```python
from build123d import *

# Parameters (mm, degrees)
SKETCH1_R                      = 20.125
BOSS_EXTRUDE1_DEPTH            = 20
SKETCH12_W                     = 21.496046148
SKETCH12_H                     = 21.496046148
CUT_EXTRUDE1_DEPTH             = 15
CUT_EXTRUDE2_START             = -18
SKETCH16_R                     = 20.125
SKETCH16_R_2                   = 19.3
CUT_EXTRUDE2_DEPTH             = 18
FILLET3_R                      = 2
M5_CLEARANCE_HOLE1_D           = 5.5
M5_CLEARANCE_HOLE1_CSINK_D     = 5.55
M5_CLEARANCE_HOLE1_CSINK_ANGLE = 90


with BuildPart() as part:
    # Sketch1 → Boss-Extrude1 (new body)
    with BuildSketch(Plane(origin=(0, 0, 0), x_dir=(1, 0, 0), z_dir=(0, 1, 0))):
        with Locations(Location((0, 0, 0), (0, 0, 270))):
            Circle(SKETCH1_R)
    extrude(amount=BOSS_EXTRUDE1_DEPTH)

    # Sketch12 → Cut-Extrude1 (cut)
    with BuildSketch(Plane.XZ):
        Rectangle(SKETCH12_W, SKETCH12_H)
    extrude(amount=-CUT_EXTRUDE1_DEPTH, mode=Mode.SUBTRACT)

    # Sketch16 → Cut-Extrude2 (cut)
    with BuildSketch(Plane(origin=(0, 20, 0), x_dir=(1, 0, 0), z_dir=(0, 1, 0)).offset(CUT_EXTRUDE2_START)):
        with Locations(Location((0, 0, 0), (0, 0, 270))):
            Circle(SKETCH16_R)
        with Locations(Location((0, 0, 0), (0, 0, 270))):
            Circle(SKETCH16_R_2, mode=Mode.SUBTRACT)
    extrude(amount=CUT_EXTRUDE2_DEPTH, mode=Mode.SUBTRACT)

    # Fillet3
    # the kernel refuses this fillet: 2 mm, written as the material it takes off along each edge
    with BuildSketch(Plane(origin=(0, 20, 0), x_dir=(0, 0, 1), z_dir=(-1, 0, 0))) as fillet3_piece_1:
        with BuildLine():
            CenterArc((19.3 - FILLET3_R, -FILLET3_R), FILLET3_R, 0, 90)
            Line((19.3 - FILLET3_R, 0), (19.3 - FILLET3_R, FILLET3_R * 0.02))
            Line((19.3 - FILLET3_R, FILLET3_R * 0.02), (19.3 + FILLET3_R * 0.02, FILLET3_R * 0.02))
            Line((19.3 + FILLET3_R * 0.02, FILLET3_R * 0.02), (19.3 + FILLET3_R * 0.02, -FILLET3_R))
            Line((19.3 + FILLET3_R * 0.02, -FILLET3_R), (19.3, -FILLET3_R))
        make_face()
    revolve(axis=Axis((0, 20, 0), (0, 1, 0)), mode=Mode.SUBTRACT)
    with BuildSketch(Plane(origin=(0, 2, 0), x_dir=(0, 0, 1), z_dir=(-1, 0, 0))) as fillet3_piece_2:
        with BuildLine():
            CenterArc((18.125, -1.618448331), FILLET3_R, 0, 54.020199403)
            Line((19.3, 0), (19.3235, 0.032368967))
            ThreePointArc((19.3235, 0.032368967), (19.7125, 0.04), (20.125, 0.04))
            Line((20.125, 0.04), (20.165, 0))
            Line((20.165, 0), (20.165, -1.618448331))
            Line((20.165, -1.618448331), (20.125, -1.618448331))
        make_face()
    revolve(axis=Axis((0, 2, 0), (0, 1, 0)), mode=Mode.SUBTRACT)

    # M5 Clearance Hole1 (through all)
    with Locations(Plane(origin=(0, 20, 0), x_dir=(1, 0, 0), z_dir=(0, 1, 0))):
        with Locations((0, 0)):
            CounterSinkHole(M5_CLEARANCE_HOLE1_D / 2, M5_CLEARANCE_HOLE1_CSINK_D / 2, counter_sink_angle=M5_CLEARANCE_HOLE1_CSINK_ANGLE)


solid = part.part
```
The listing builds one solid part. Answer for the finished solid, in the listing's coordinates (mm). A direction names the side the tool comes from. Coordinates: 2 decimals unless noted, no trailing zeros. Loops run counter-clockwise (first coordinate to the right, second up) from the corner with the lowest first, then second, coordinate; pieces in that order, holes last. Notation, with made-up numbers: M -1,42.5 L 40,42.5 A28 ccw 40,73.5 Z; hole C 60.25,-7.5 d5. An arc over 180 degrees is marked long. Answer as a JSON object with one key per item and string values. Group by question number.
Item 1: Section B-B (x = 0) is taken. Write down the section's boundary in (y, z) (3 decimals), and give its area (3 significant figures).
Item 2: Each of these flat-tipped pins is pushed along its axis until it touches: P1, Ø5, axis at x = 7.5, y = 5.5, coming from the +Z side; P2, Ø12, axis at y = 5.5, z = 1, coming from the +X side (3 decimals); P3, Ø3, axis at y = 15, z = 15, coming from the +X side. Where does it stop, or does it pass through?
Item 3: Determine the mould class of faces 1 (the face through (-10.748, 7, 0)), 2 (the face through (0, 20, 4)), 3 (the face through (10.748, 7, 0)), 4 (the face through (6.045, 0.188, 19.196)) for opening direction Z: +Z half, -Z half, draft (parallel to the pull), parting line (faces both ways), or undercut.
Item 4: Section D-D (y = 15.75) is taken. Write down the section's boundary in (x, z), and give its area (3 significant figures).
Item 5: Consider L1, parallel to X at y = 8, z = 0.5; L2, parallel to X at y = 10.75, z = 2; L3, parallel to Y at x = 10, z = -4. Determine where each line is inside the solid, lowest interval first.
Item 6: Section A-A (z = 0) is taken. Write down the section's boundary in (x, y) (3 decimals).
Item 7: Which of the six approach directions +Z, -Z, +X, -X, +Y, -Y give full straight-line access (tool end or side, diameter ignored) to faces 5 (the face through (0.596, 17.453, 2.685)), 6 (the face through (0, 7, 10.748)), 7 (the face through (19.136, 9.888, -2.512))?
Item 8: Section C-C (y = 9) is taken. Write down the section's boundary in (x, z), and give its area (3 significant figures).
Solved:
{
 "1": {"outline": "M 0,-20.125 L 0.382,-20.125 A2 ccw 2,-19.3 L 18,-19.3 A2 ccw 20,-17.3 L 20,-2.775 L 19.975,-2.75 L 15,-2.75 L 15,-10.748 L 0,-10.748 Z; M 0,10.748 L 15,10.748 L 15,2.75 L 19.975,2.75 L 20,2.775 L 20,17.3 A2 ccw 18,19.3 L 2,19.3 A2 ccw 0.382,20.125 L 0,20.125 Z", "area": "423 mm2"},
 "2": {"P1": "stops at z = 18.64", "P2": "stops at x = 20.125", "P3": "stops at x = 13.79"},
 "3": {"face 1": "undercut", "face 2": "draft", "face 3": "undercut", "face 4": "parting line"},
 "4": {"outline": "C 0,0 d38.6; hole C 0,0 d5.5", "area": "1,150 mm2"},
 "5": {"L1": "x = -19.29 to -10.75, 10.75 to 19.29", "L2": "x = -19.2 to -10.75, 10.75 to 19.2", "L3": "y = 15 to 20"},
 "6": {"outline": "M -20.125,0 L -10.748,0 L -10.748,15 L -2.75,15 L -2.75,19.975 L -2.775,20 L -17.3,20 A2 ccw -19.3,18 L -19.3,2 A2 ccw -20.125,0.382 Z; M 2.75,15 L 10.748,15 L 10.748,0 L 20.125,0 L 20.125,0.382 A2 ccw 19.3,2 L 19.3,18 A2 ccw 17.3,20 L 2.775,20 L 2.75,19.975 Z"},
 "7": {"face 5": "+Y, -Y", "face 6": "-Y", "face 7": "+Y"},
 "8": {"outline": "C 0,0 d38.6; hole M -10.75,-10.75 L 10.75,-10.75 L 10.75,10.75 L -10.75,10.75 Z", "area": "708 mm2"}
}
